The model under review builds one solid part; all positions refer to its coordinate system, in mm. A direction names the side the tool comes from. Coordinates: 2 decimals unless noted, no trailing zeros. Order: outer loops, then holes, each group sorted by start corner. A loop starts at its lowest first (then second) coordinate and runs counter-clockwise, first axis right, second up.
from build123d import *

# Parameters (mm, degrees)
F1_DEPTH  = 10
F2_R      = 1.6
F3_DEPTH  = 3
F3_FACE_R = 1.6
F4_DEPTH  = 25
F5_R      = 1.6
F6_DEPTH  = 3
F6_FACE_R = 1.6
F7_DEPTH  = 25


with BuildPart() as f1:
    # F0 (on Front) → F1 (new body)
    with BuildSketch(Plane.XZ):
        Polygon((-14, 0), (0, 0), (0, 14), (-4.75, 14), (-4.75, 4.75), (-14, 4.75), align=None)
    extrude(amount=F1_DEPTH)

    # F2 (on face) → F3 (cut)
    with BuildSketch(Plane(origin=(-4.75, 0, 0), x_dir=(0, -1, 0), z_dir=(-1, 0, 0))):
        Polygon((2, 11.107051), (2, 7.642949), (5, 5.910898), (8, 7.642949), (8, 11.107051), (5, 12.839102), align=None)
        with Locations((5, 9.375)):
            Circle(F2_R, mode=Mode.SUBTRACT)
    extrude(amount=-F3_DEPTH, mode=Mode.SUBTRACT)

    # F3_face (on face) → F4 (cut)
    with BuildSketch(Plane(origin=(-4.75, -5, 9.375), x_dir=(0, -1, 0), z_dir=(-1, 0, 0))):
        Circle(F3_FACE_R)
    extrude(amount=-F4_DEPTH, mode=Mode.SUBTRACT)

    # F5 (on face) → F6 (cut)
    with BuildSketch(Plane.XY.offset(4.75)):
        Polygon((-11.107051, -8), (-7.642949, -8), (-5.910898, -5), (-7.642949, -2), (-11.107051, -2), (-12.839102, -5), align=None)
        with Locations((-9.375, -5)):
            Circle(F5_R, mode=Mode.SUBTRACT)
    extrude(amount=-F6_DEPTH, mode=Mode.SUBTRACT)

    # F6_face (on face) → F7 (cut)
    with BuildSketch(Plane(origin=(-9.375, -5, 4.75), x_dir=(1, 0, 0), z_dir=(0, 0, 1))):
        Circle(F6_FACE_R)
    extrude(amount=-F7_DEPTH, mode=Mode.SUBTRACT)


solid = f1.part
(1) Consider section A-A (x = -3.5). Give the boundary of the cut face in (y, z).
(2) Wall thickness on line 1 (Y direction, x = -2, z = 11); line 2 (Z direction, x = -1.15, y = -5) (3 decimals); line 3 (Z direction, x = -8.75, y = -7.5): over which ranges is each line inside the solid? List them lowest first.
(3) The part is to be moulded in two halves that separate along Z. For faces 4 (the face through (-7, -5, 0)), 5 (the face through (-3.27, -3.48, 6.79)), 6 (the face through (-7.9, -3.6, 1.75)), 7 (the face through (-11.985, -6.479, 3.271)), say which applies: +Z half, -Z half, draft (parallel to the pull), parting line (faces both ways), or undercut.
(4) Consider section D-D (x = -8). Give the boundary of the cut face in (y, z), then the cut area to 3 significant figures.
(5) Consider section B-B (y = -4.25). Give the boundary of the cut face in (x, z), then the cut area to 3 significant figures.
(6) Insertion check: pin 1 Ø1.8 at (x, y) = (-7.5, -5) entering from +Z; pin 2 Ø4.5 at (y, z) = (-5.5, 9) entering from -X; pin 3 Ø1 at (x, y) = (-5.5, -6) entering from +Z. Each pin has a flat end and moves straight along its axis. Give the tip position at first contact, or say it passes through.
(7) Tool access review of faces 1 (the face through (-3, -8, 9)), 2 (the face through (-11.96, -3.48, 3.27)), 3 (the face through (-6, -4, 4.75)): name each direction out of +Z, -Z, +X, -X, +Y, -Y from which nothing blocks a thin tool from reaching the whole face with its end or side.
(8) Consider section C-C (z = 2.5). Give the boundary of the cut face in (x, y), then the cut area to 3 significant figures.
Findings:
1. outline: (-10, 0) - (0, 0) - (0, 14) - (-10, 14) - close; hole (-8, 7.64) - (-5, 5.91) - (-2, 7.64) - (-2, 11.11) - (-5, 12.84) - (-8, 11.11) - close
2. line 1: y = -10 to -8, -2 to 0
2. line 2: z = 0 to 7.775, 10.975 to 14
2. line 3: z = 0 to 1.75
3. face 4: -Z half
3. face 5: undercut
3. face 6: +Z half
3. face 7: draft
4. outline: (-10, 0) - (-5.82, 0) - (-5.82, 1.75) - (-8, 1.75) - (-8, 4.75) - (-10, 4.75) - close; (-4.18, 0) - (0, 0) - (0, 4.75) - (-2, 4.75) - (-2, 1.75) - (-4.18, 1.75) - close
4. area: 26.6 mm2
5. outline: (-14, 0) - (-10.79, 0) - (-10.79, 1.75) - (-12.41, 1.75) - (-12.41, 4.75) - (-14, 4.75) - close; (-7.96, 0) - (0, 0) - (0, 7.96) - (-1.75, 7.96) - (-1.75, 6.34) - (-4.75, 6.34) - (-4.75, 4.75) - (-6.34, 4.75) - (-6.34, 1.75) - (-7.96, 1.75) - close; (-4.75, 12.41) - (-1.75, 12.41) - (-1.75, 10.79) - (0, 10.79) - (0, 14) - (-4.75, 14) - close
5. area: 64.2 mm2
6. pin 1: stops at z = 1.75
6. pin 2: stops at x = -1.75
6. pin 3: stops at z = 4.75
7. face 1: -X
7. face 2: +Z
7. face 3: +Z, -X, +Y, -Y
8. outline: (-14, -10) - (0, -10) - (0, 0) - (-14, 0) - close; hole (-12.84, -5) - (-11.11, -8) - (-7.64, -8) - (-5.91, -5) - (-7.64, -2) - (-11.11, -2) - close
8. area: 109 mm2
